Check sheet for the modelled part. Datum: model origin and axes. Units: mm. A direction names the side the tool comes from. Coordinates: 2 decimals unless noted, no trailing zeros. One line per item, written item: value. Start each with the question number.
1) Set-up check for faces 1 (the flat face through (-48.84, -36.493, 30.303)), 2 (the flat face through (-48.26, 34, 22)), 3 (the flat face through (-45.329, -41.487, 34.707)): record each of +Z, -Z, +X, -X, +Y, -Y from which the full face is reachable in a straight line by a thin tool's end or side.
2) Draft check along Z on faces 4 (the flat face through (-45.33, 41.51, 34.64)), 5 (the flat face through (-53.34, 34, 32)), 6 (the flat face through (-48.84, 36.28, 30.23)). Enter one of: +Z half, -Z half, draft (parallel to the pull), parting line (faces both ways), or undercut.
3) Scan lines: line 1 along Y through (x, z) = (-1, 17.5); line 2 along Y through (x, z) = (-27, 36.5); line 3 along X through (y, z) = (0.5, 24). Record each from-to range of solid material in increasing order. Write a range as [from, to].
4) Gauge pin test, flat ends, axial feed: P1, Ø5, axis at y = 30.5, z = 30.5, coming from the -X side; P2, Ø1.5, axis at x = 45, y = 24.5, coming from the +Z side; P3, Ø4, axis at y = 14.5, z = 23.5, coming from the +X side. Record the tip position at first contact, or that the pin passes through.
```python
from build123d import *

# Parameters (mm, degrees)
F0_R     = 56.608289
F1_DEPTH = 71.12
F2_R     = 30.48
F3_W     = 8.632271
F3_H     = 8.368614
F4_DEPTH = 48.26
F6_DEPTH = 53.34


with BuildPart() as f1:
    # F0 (on Top) → F1 (new body)
    with BuildSketch(Plane.XY):
        Circle(F0_R)
    extrude(amount=F1_DEPTH)

    # F2
    f2_edges = [f1.edges().sort_by_distance(p)[0] for p in [
        (-56.608289, 0, 71.12),
    ]]
    fillet(f2_edges, radius=F2_R)

    # F3 (on Right) → F4 (join)
    with BuildSketch(Plane.YZ):
        with Locations((34.341916, 21.801914)):
            Rectangle(F3_W, F3_H)
        with Locations((-34.341916, 21.801914)):
            Rectangle(F3_W, F3_H)
    extrude(amount=-F4_DEPTH)

    # F5 (on Right) → F6 (join)
    with BuildSketch(Plane.YZ):
        Polygon((42.371512, 32.300244), (40.627647, 37.047431), (25.372822, 31.443618), (26.978905, 27.071502), align=None)
        Polygon((-26.978905, 27.071502), (-25.372822, 31.443618), (-40.627647, 37.047431), (-42.371512, 32.300244), align=None)
    extrude(amount=-F6_DEPTH)


solid = f1.part
```
Answers:
1. face 1: -X, -Y
1. face 2: -Z, -X, +Y
1. face 3: +Z, -X, -Y
2. face 4: +Z half
2. face 5: draft
2. face 6: undercut
3. line 1: y = [-56.6, 56.6]
3. line 2: y = [-49.75, 49.75]
3. line 3: x = [-56.61, 56.61]
4. P1: stops at x = -53.34
4. P2: stops at z = 58.96
4. P3: stops at x = 55.21
